Here's how the part is built. I have some questions about the finished solid (model axes, mm). A direction names the side the tool comes from. Coordinates: 2 decimals unless noted, no trailing zeros. Write each loop counter-clockwise with the first axis right and the second up, starting at its lowest first coordinate (ties: lowest second). Pieces come first, ordered by that corner, then holes. Notation, with made-up numbers: (-9.5, 85.5) - (29.5, 85.5) arc R10 ccw to (29.5, 97.5) - close; hole circle Ø8 at (49.25, 53). An arc over 180 degrees is marked (long way). Answer in a Markdown table with one row per item. Add a question column.
Item 1: Imagine slicing it at C-C (x = 20). Please give me the cut outline in (y, z).
Item 2: Imagine slicing it at B-B (z = 5.5). Please give me the cut outline in (x, y), plus the area to 3 significant figures.
Item 3: Imagine slicing it at A-A (x = 0). Please give me the cut outline in (y, z).
Item 4: We'd pull the mould along X, two halves only. Please class faces 6 (the face through (25, 0, 3)), 7 (the face through (5, 1, 7)), 8 (the face through (1.523, -34.384, 5.028)): +X half, -X half, draft (parallel to the pull), parting line (faces both ways), or undercut.
Item 5: Which directions (+Z, -Z, +X, -X, +Y, -Y) give clear straight access to the entire face, cutting with the end or side of a thin tool? Please do faces 1 (the face through (2.986, -1.756, 5.521)), 2 (the face through (-10, -31, 4)), 3 (the face through (10, -32, 4)), 4 (the face through (0.29, 2.23, 1.97)), 5 (the face through (10, 31, 4)).
Item 6: If I drill on probe 1 along Y at (x, z) = (0, 5.9); probe 2 along Y at (x, z) = (0, 1.15); probe 3 along X at (y, z) = (23.5, 4), over which ranges is the centre line in solid material (lowest first)? Write a range as from..to.
Item 7: Imagine slicing it at D-D (y = -19). Please give me the cut outline in (x, z).
Item 8: I'm going to push flat-ended pins straight in: pin 1 (3 mm diameter, centred on x = -16.5, z = 4.5, fed in from +Y); pin 2 (1.5 mm diameter, centred on x = 11, z = 4.5, fed in from +Y); pin 3 (2 mm diameter, centred on y = 27.5, z = 2.5, fed in from -X). Where does each tip first touch, or does it pass through?
from build123d import *

# Parameters (mm, degrees)
SKETCH1_R                                           = 25
BOSS_EXTRUDE1_DEPTH                                 = 7
BOSS_EXTRUDE2_DEPTH                                 = 7
CSK_FOR_M6_COUNTERSUNK_FLAT_HEAD_SCREW2_D           = 6.6
CSK_FOR_M6_COUNTERSUNK_FLAT_HEAD_SCREW2_CSINK_D     = 12.6
CSK_FOR_M6_COUNTERSUNK_FLAT_HEAD_SCREW2_CSINK_ANGLE = 90
CUT_EXTRUDE1_DEPTH                                  = 3
M4_CLEARANCE_HOLE1_D                                = 4.5
M4_CLEARANCE_HOLE1_DEPTH                            = 10
M4_CLEARANCE_HOLE1_TIP                              = 1.351936393
CIRPATTERN1_COUNT                                   = 2


with BuildPart() as part:
    # Sketch1 → Boss-Extrude1 (new body)
    with BuildSketch(Plane.XY):
        Circle(SKETCH1_R)
    extrude(amount=BOSS_EXTRUDE1_DEPTH)

    # Sketch2 → Boss-Extrude2 (add)
    with BuildSketch(Plane.XY.offset(7)):
        with BuildLine():
            Line((-10, -40), (10, -40))
            Line((10, -40), (10, -22.912878475))
            ThreePointArc((10, -22.912878475), (0, -25), (-10, -22.912878475))
            Line((-10, -22.912878475), (-10, -40))
        make_face()
    boss_extrude2 = extrude(amount=-BOSS_EXTRUDE2_DEPTH)

    # CSK for M6 Countersunk Flat Head Screw2 (through all)
    with Locations(Plane(origin=(0, 0, 0), x_dir=(-1, 0, 0), z_dir=(0, 0, -1))):
        with Locations((0, -31.456439237)):
            csk_for_m6_countersunk_flat_head_screw2 = CounterSinkHole(CSK_FOR_M6_COUNTERSUNK_FLAT_HEAD_SCREW2_D / 2, CSK_FOR_M6_COUNTERSUNK_FLAT_HEAD_SCREW2_CSINK_D / 2, counter_sink_angle=CSK_FOR_M6_COUNTERSUNK_FLAT_HEAD_SCREW2_CSINK_ANGLE)

    # Sketch10 → Cut-Extrude1 (cut)
    with BuildSketch(Plane.XY.offset(7)):
        Polygon((4, 0), (2, 3.464101615), (-2, 3.464101615), (-4, 0), (-2, -3.464101615), (2, -3.464101615), align=None)
    extrude(amount=-CUT_EXTRUDE1_DEPTH, mode=Mode.SUBTRACT)

    # M4 Clearance Hole1
    with Locations(Plane.XY.offset(4)):
        with Locations((0, 0)):
            Hole(M4_CLEARANCE_HOLE1_D / 2, depth=M4_CLEARANCE_HOLE1_DEPTH)
            with Locations((0, 0, -(M4_CLEARANCE_HOLE1_DEPTH + M4_CLEARANCE_HOLE1_TIP / 2))):  # 118° drill point
                Cone(0, M4_CLEARANCE_HOLE1_D / 2, M4_CLEARANCE_HOLE1_TIP, mode=Mode.SUBTRACT)

    # CirPattern1: Boss-Extrude2, CSK for M6 Countersunk Flat Head Screw2 ×2 about axis
    cirpattern1_axis = Axis((0, 0, 0), (0, 0, 1))
    for i in range(1, CIRPATTERN1_COUNT):
        add(boss_extrude2.rotate(cirpattern1_axis, i * 360 / CIRPATTERN1_COUNT))
        add(csk_for_m6_countersunk_flat_head_screw2.rotate(cirpattern1_axis, i * 360 / CIRPATTERN1_COUNT), mode=Mode.SUBTRACT)


solid = part.part
Here are the results:
| question | item | result |
|---|---|---|
| 1 | outline | (-15, 0) - (15, 0) - (15, 7) - (-15, 7) - close |
| 2 | outline | (-10, -40) - (10, -40) - (10, -22.91) arc R25 ccw to (10, 22.91) - (10, 40) - (-10, 40) - (-10, 22.91) arc R25 ccw to (-10, -22.91) - close; hole (-4, 0) - (-2, -3.46) - (2, -3.46) - (4, 0) - (2, 3.46) - (-2, 3.46) - close; hole circle Ø6.6 at (0, -31.46); hole circle Ø6.6 at (0, 31.46) |
| 2 | area | 2,480 mm2 |
| 3 | outline | (-40, 0) - (-37.76, 0) - (-34.76, 3) - (-34.76, 7) - (-40, 7) - close; (-28.16, 3) - (-25.16, 0) - (-2.25, 0) - (-2.25, 4) - (-3.46, 4) - (-3.46, 7) - (-28.16, 7) - close; (2.25, 0) - (25.16, 0) - (28.16, 3) - (28.16, 7) - (3.46, 7) - (3.46, 4) - (2.25, 4) - close; (34.76, 3) - (37.76, 0) - (40, 0) - (40, 7) - (34.76, 7) - close |
| 4 | face 6 | +X half |
| 4 | face 7 | draft |
| 4 | face 8 | undercut |
| 5 | face 1 | +Z |
| 5 | face 2 | +Z, -Z, -X, -Y |
| 5 | face 3 | +Z, -Z, +X, -Y |
| 5 | face 4 | +Z, -Z |
| 5 | face 5 | +Z, -Z, +X, +Y |
| 6 | probe 1 | y = -40..-34.76, -28.16..-3.46, 3.46..28.16, 34.76..40 |
| 6 | probe 2 | y = -40..-36.61, -26.31..-2.25, 2.25..26.31, 36.61..40 |
| 6 | probe 3 | x = -10..10 |
| 7 | outline | (-16.25, 0) - (16.25, 0) - (16.25, 7) - (-16.25, 7) - close |
| 8 | pin 1 | stops at y = 20 |
| 8 | pin 2 | stops at y = 22.8 |
| 8 | pin 3 | stops at x = -10 |
